Could you check a few things on this drawing? It's one solid part, dimensions in mm from its lowest x, y, z. Give positions to 0.01 mm unless a question says otherwise; leave off trailing zeros. Loops run counter-clockwise (first coordinate to the right, second up) from the corner with the lowest first, then second, coordinate; pieces in that order, holes last. Notation, with made-up numbers: (89, -36.5) - (93, -36.5) arc R36 ccw to (93, 2.5) - close; hole circle Ø11 at (39, -33). An arc over 180 degrees is marked (long way). Return JSON: item names as keys, results as strings. Group by question number.
(1) If we section it at B-B (x = 131): Please give me the cut outline in (y, z), then the cut area to 3 significant figures.
(2) If we section it at C-C (z = 383): Please give me the cut outline in (x, y).
(3) I need wall thicknesses on probe 1 along Z at (x, y) = (157.5, 7.5); probe 2 along Z at (x, y) = (250, 3.75); probe 3 along X at (y, z) = (11, 303.5). Which ranges of each line are inside material? Lowest first, please. Write a range as [from, to].
(4) For P1, Ø5, axis at y = 9.5, z = 278, coming from the -X side; P2, Ø3, axis at x = 197, y = 4.5, coming from the +Z side; P3, Ø4, axis at x = 143, y = 9, coming from the +Z side, each with a flat end and sliding along its axis, tell me the tip position at first contact or that it passes through.
(5) If we section it at A-A (y = 8): Please give me the cut outline in (x, z), then the cut area to 3 significant figures.
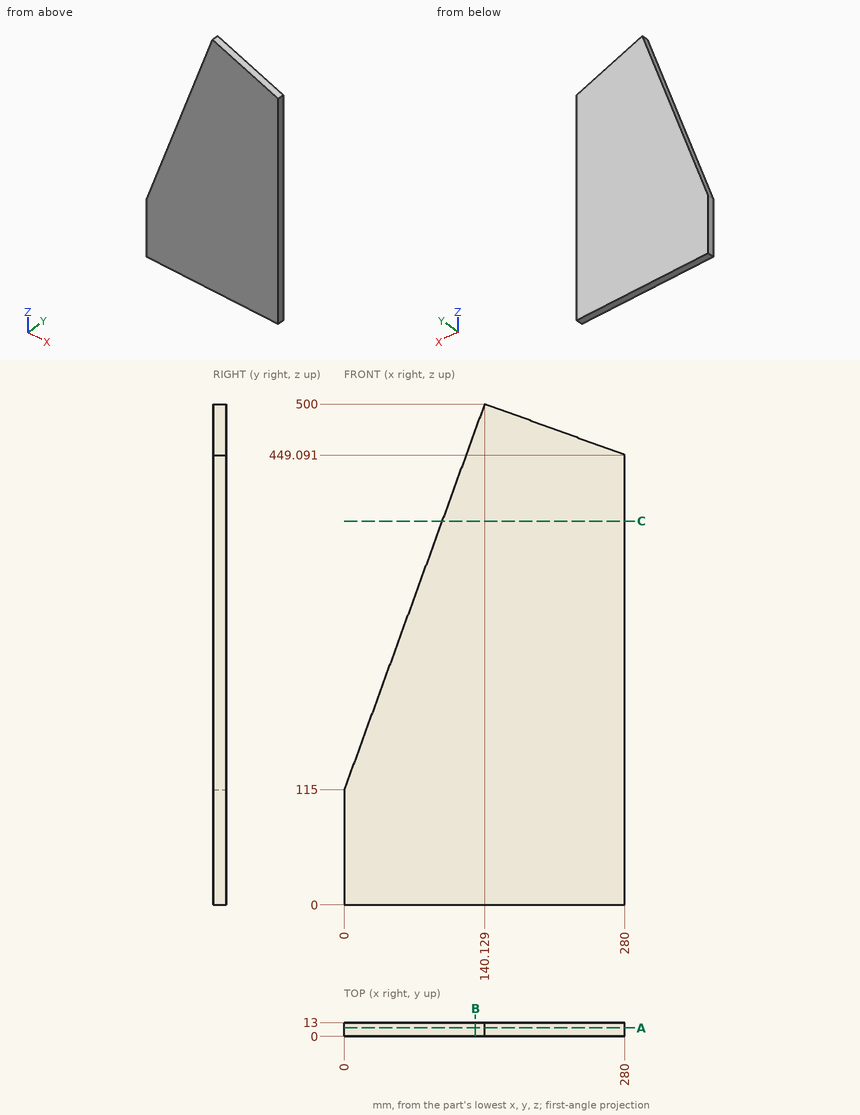
Values:
{
 "1": {"outline": "(0, 0) - (13, 0) - (13, 474.92) - (0, 474.92) - close", "area": "6,170 mm2"},
 "2": {"outline": "(97.54, 0) - (280, 0) - (280, 13) - (97.54, 13) - close"},
 "3": {"probe 1": "[0, 493.68]", "probe 2": "[0, 460.01]", "probe 3": "[68.61, 280]"},
 "4": {"P1": "x = 58.42", "P2": "z = 479.85", "P3": "z = 499.68"},
 "5": {"outline": "(0, 0) - (280, 0) - (280, 449.09) - (140.13, 500) - (0, 115) - close", "area": "109,000 mm2"}
}
